Geometry check sheet. Reference: the model listing, model coordinates, mm. A direction names the side the tool comes from. Give positions to 0.01 mm unless a question says otherwise; leave off trailing zeros. Write each loop counter-clockwise with the first axis right and the second up, starting at its lowest first coordinate (ties: lowest second). Pieces come first, ordered by that corner, then holes. Notation, with made-up numbers: (40.25, -37.5) -> (75.25, -37.5) arc R37 cw to (75.25, 0.5) -> close; hole circle Ø2 at (-40, -18). An arc over 180 degrees is marked (long way). One line per item, written item: value.
Solid Edge part; units mm, degrees
sketch "Sketch1" plane through (0, 0, 0) normal (0, 0, 1) x (1, 0, 0)
  line L0 (-34, -10) -> (34, -10)
  line L1 (34, -10) -> (34, 10)
  line L2 (34, 10) -> (-34, 10)
  line L3 (-34, 10) -> (-34, -10)
  line L4 (-35, -15) -> (35, -15)
  line L5 (40, -10) -> (35, -15)
  line L6 (40, -10) -> (40, 10)
  line L7 (35, 15) -> (40, 10)
  line L8 (35, 15) -> (-35, 15)
  line L9 (-35, 15) -> (-40, 10)
  line L10 (-40, 10) -> (-40, -10)
  line L11 (-40, -10) -> (-35, -15)
extrude "Protrusion1" add sketch "Sketch1" along normal blind 75
sketch "Sketch2" plane through (0, 0, 75) normal (0, 0, 1) x (1, 0, 0)
  line L0 (-34.8, -0.975) -> (35.15, -0.975)
  line L1 (35.15, -0.975) -> (35.15, 0.975)
  line L2 (35.15, 0.975) -> (-34.8, 0.975)
  line L3 (-34.8, 0.975) -> (-34.8, -0.975)
extrude "Wycięcie_1" cut sketch "Sketch2" against normal blind 68
chamfer "Faza_1" distance 0.5 angle 45 4 edges at (-34, -0.975, 41) (-34, 0.975, 41) (34, -0.975, 41) (34, 0.975, 41)
sketch "Sketch3" plane through (0, 15, 32.5) normal (0, 1, 0) x (-1, 0, 0)
  line L0 (-35, 17.5) -> (-5, 17.5)
  line L1 (-35, 42.5) -> (-35, 17.5)
  line L2 (-35, 42.5) -> (0, 42.5)
  line L3 (-5, 17.5) -> (0, 42.5)
extrude "Cutout1" cut sketch "Sketch3" against normal up to next
sketch "Sketch4" plane through (0, 15, 32.5) normal (0, 1, 0) x (-1, 0, 0)
  line L0 (-35, -32.5) -> (35, -32.5)
  line L1 (35, -32.5) -> (26.3397, -17.5)
  line L2 (26.3397, -17.5) -> (-26.3397, -17.5)
  line L3 (-35, -32.5) -> (-26.3397, -17.5)
extrude "Cutout2" cut sketch "Sketch4" against normal up to vertex (25 mm away)
sketch "Sketch5" plane through (0, 15, 32.5) normal (0, 1, 0) x (0, 0, 1)
  line L0 (-10, -29.027) -> (35, -29.027)
  line L1 (35, -29.027) -> (35, -4.027)
  line L2 (35, -4.027) -> (-10, -4.027)
  line L3 (-10, -4.027) -> (-10, -29.027)
extrude "Wycięcie_4" cut sketch "Sketch5" against normal blind 1
chamfer "Faza_3" distance 1 angle 45 4 edges at (-4.027, 15, 45) (-16.527, 15, 22.5) (-29.027, 15, 45) (-16.527, 15, 67.5)
chamfer "Chamfer1" [suppressed]
chamfer "Faza_7" [suppressed]
chamfer "Faza_8" distance 2 angle 45 1 edges at (0, 12.5, 75)
1) Scan lines: probe 1 along Y at (x, z) = (-13, 48); probe 2 along Y at (x, z) = (18, 24.5); probe 3 along X at (y, z) = (2.5, 13.5). Record each from-to range of solid material in increasing order.
Verdict:
probe 1: -15 to -10, 10 to 14
probe 2: -15 to -10, 10 to 15
probe 3: -40 to -34, 34 to 40
2) Mould release check, pull along X, two halves, no side actions. Record for faces 1 (the flat face through (-38, -12, 37)), 2 (the flat face through (0, 13, 15)), 3 (the flat face through (0, -15, 37)): released by +X, released by -X, zero draft, split by the parting line, or undercut.
Verdict:
face 1: released by -X
face 2: undercut
face 3: zero draft
3) Sectioned sample at C-C on y = 8.5. Record the cut outline in (x, z), plus the area to 3 significant figures.
Verdict:
outline: (-40, 0) -> (-35, 0) -> (-34, 1.73) -> (-34, 75) -> (-40, 75) -> close; (34, 1.73) -> (35, 0) -> (40, 0) -> (40, 75) -> (35, 75) -> (35, 50) -> (34, 50) -> close
area: 873 mm^2
4) Sectioned sample at A-A on x = 1.5. Record the cut outline in (y, z).
Verdict:
outline: (-15, 0) -> (-10, 0) -> (-10, 75) -> (-15, 75) -> close; (10, 15) -> (15, 15) -> (15, 67.5) -> (10, 67.5) -> close
5) Depth check by flat-ended pin: pin 1 Ø11 at (x, y) = (23, 8.5) entering from +Z; pin 2 Ø2 at (x, z) = (30, 54.5) entering from +Y; pin 3 Ø4 at (x, y) = (11.5, 13) entering from -Z. Enter the tip coordinate at first touch or a pass-through.
Verdict:
pin 1: z = 50
pin 2: y = -10
pin 3: z = 15
6) Tool access check on faces 4 (the flat face through (-0.821, 12.535, 74.033)), 5 (the flat face through (0, -10, 37)), 6 (the flat face through (-31.65, 10.89, 5.8)), 7 (the flat face through (35.15, 0, 41)). Record the directions out of +Z, -Z, +X, -X, +Y, -Y that give a thin tool (end or side, any length) a straight path to the whole face; none if there is none.
Verdict:
face 4: +Z, +Y
face 5: +Z, -Z
face 6: -Z, +Y
face 7: +Z
